from build123d import *

# Parameters (mm, degrees)
F0_W     = 250
F0_H     = 20
F1_DEPTH = 550
F3_DEPTH = 12.5


with BuildPart() as f1:
    # F0 (on Top) → F1 (new body)
    with BuildSketch(Plane.XY):
        Rectangle(F0_W, F0_H)
    extrude(amount=F1_DEPTH)

    # F2 (on Front) → F3 (join, symmetric)
    with BuildSketch(Plane.XZ):
        Polygon((75, 0), (75, -75), (-75, -75), (-75, 0), (-125.045896, 0), (-350, -200), (350, -200), (124.919437, 0), align=None)
    extrude(amount=F3_DEPTH, both=True)


solid = f1.part
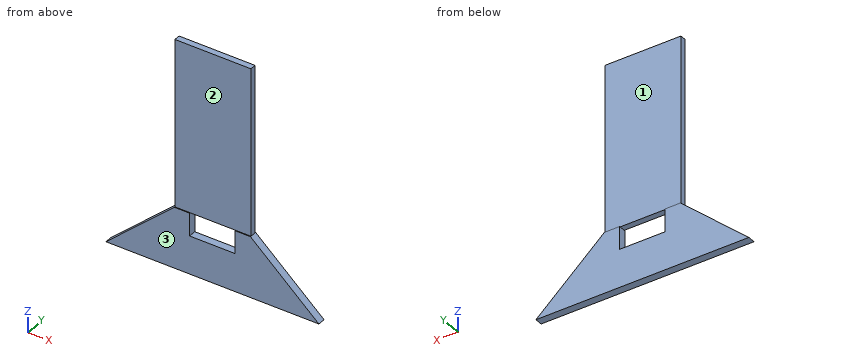
Build history of the part. All positions in model axes, mm. Face numbers are marked on the shaded views. A direction names the side the tool comes from. Coordinates: 2 decimals unless noted, no trailing zeros. Order: outer loops, then holes, each group sorted by start corner. A loop starts at its lowest first (then second) coordinate and runs counter-clockwise, first axis right, second up. Notation, with made-up numbers: (0, -28) - (24, -28) arc R30 cw to (24, -4) - close; hole circle Ø1 at (-32, 39.25). An arc over 180 degrees is marked (long way). Write item = value, one per line. Start each with the question number.
1) Saw through at C-C on z = 264. Write the cut outline in (x, y).
2) 3-axis set-ups, long thin cutter, end or side, ignore diameter. For the marked faces 1, 2 and 3: which of +Z, -Z, +X, -X, +Y, -Y reach the whole face in a straight line?
3) Saw through at A-A on y = 4. Write the cut outline in (x, z).
4) Flat gauge pins, fed straight in: pin 1 Ø0.8 at (x, y) = (109, -10.5) entering from +Z; pin 2 Ø10 at (x, y) = (170, -2) entering from +Z; pin 3 Ø6 at (x, z) = (127.5, 360.5) entering from -Y. Where does each tip first touch, or does it go through?
5) Saw through at D-D on x = -207. Write the cut outline in (y, z).
6) Saw through at B-B on x = -105. Write the cut outline in (y, z).
7) Wall check: line 1 along Z through (x, y) = (11.5, -9.75); line 2 along Y through (x, z) = (-13, 120.5); line 3 along X through (y, z) = (4.25, 285). Give the ranges that are in metal, low to high. Write a range as from..to.
From the geometry:
q1.outline = (-125, -10) - (125, -10) - (125, 10) - (-125, 10) - close
q2.face_1 = +Z, +X, -X, +Y
q2.face_2 = +Z, +X, -X, -Y
q2.face_3 = +Z, -Z, +X, -X, -Y
q3.outline = (-350, -200) - (350, -200) - (124.92, 0) - (125, 0) - (125, 550) - (-125, 550) - (-125, 0) - (-125.05, 0) - close; hole (-75, -75) - (75, -75) - (75, 0) - (-75, 0) - close
q4.pin_1 = 0
q4.pin_2 = -35.61
q4.pin_3 = -10
q5.outline = (-12.5, -200) - (12.5, -200) - (12.5, -72.86) - (-12.5, -72.86) - close
q6.outline = (-12.5, -200) - (12.5, -200) - (12.5, 0) - (10, 0) - (10, 550) - (-10, 550) - (-10, 0) - (-12.5, 0) - close
q7.line_1 = -200..-75, 0..550
q7.line_2 = -10..10
q7.line_3 = -125..125
